Verification items for the finished model (mm, model axes). Face numbers are marked on the shaded views. A direction names the side the tool comes from. Round coordinates to 2 decimals unless told otherwise and drop trailing zeros. Order: outer loops, then holes, each group sorted by start corner. A loop starts at its lowest first (then second) coordinate and runs counter-clockwise, first axis right, second up. Notation, with made-up numbers: M -27,-23.5 L 26,-23.5 A38 cw 26,15.5 Z; hole C -9.75,-28.5 d3. An arc over 180 degrees is marked long. Return JSON: item names as keys, results as strings. Group by question number.
from build123d import *

# Parameters (mm, degrees)
F0_R      = 12.5
F1_DEPTH  = 40
F3_W      = 45
F3_H      = 200
F4_DEPTH  = 20
F5_W      = 35
F5_H      = 80
F6_DEPTH  = 25
F9_W      = 45
F9_H      = 10
F10_DEPTH = 1
F11_W     = 45
F11_H     = 10
F12_DEPTH = 1
F15_DEPTH = 2
F17_R     = 2.5
F18_DEPTH = 20.001


with BuildPart() as f1:
    # F0 (on Front) → F1 (new body)
    with BuildSketch(Plane.XZ):
        Circle(F0_R)
    extrude(amount=F1_DEPTH)

    # F3 (on offset) → F4 (join)
    with BuildSketch(Plane.XZ.offset(10)):
        Rectangle(F3_W, F3_H)
    extrude(amount=-F4_DEPTH)

    # F5 (on face) → F6 (cut)
    with BuildSketch(Plane(origin=(0, 10, 0), x_dir=(-1, 0, 0), z_dir=(0, 1, 0))):
        with Locations((0, 55)):
            Rectangle(F5_W, F5_H)
        with Locations((0, -55)):
            Rectangle(F5_W, F5_H)
    extrude(amount=-F6_DEPTH, mode=Mode.SUBTRACT)

    # F9 (on offset) → F10 (join)
    with BuildSketch(Plane.XY.offset(80)):
        with Locations((0, -5)):
            Rectangle(F9_W, F9_H)
    extrude(amount=-F10_DEPTH)

    # F11 (on offset) → F12 (join)
    with BuildSketch(Plane.XY.offset(-80)):
        with Locations((0, -5)):
            Rectangle(F11_W, F11_H)
    extrude(amount=F12_DEPTH)


with BuildPart() as f15:
    # F14 (on offset) → F15 (new body)
    with BuildSketch(Plane.XZ.offset(5)):
        with BuildLine():
            Line((-5, 88), (-5, 80))
            Line((-5, 80), (5, 80))
            Line((5, 80), (5, 88))
            ThreePointArc((5, 88), (0, 93), (-5, 88))
        make_face()
        with BuildLine():
            Line((5, -80), (-5, -80))
            Line((-5, -80), (-5, -88))
            ThreePointArc((-5, -88), (0, -93), (5, -88))
            Line((5, -88), (5, -80))
        make_face()
    extrude(amount=-F15_DEPTH)


with BuildPart() as f1_1:
    add(f1.part)

    # F16: union F15
    add(f15.part)

    # F17 (on face) → F18 (cut, through all)
    with BuildSketch(Plane.XZ.offset(10)):
        with Locations((0, -88)):
            Circle(F17_R)
        with Locations((0, 88)):
            Circle(F17_R)
    extrude(amount=-F18_DEPTH, mode=Mode.SUBTRACT)


solid = f1_1.part
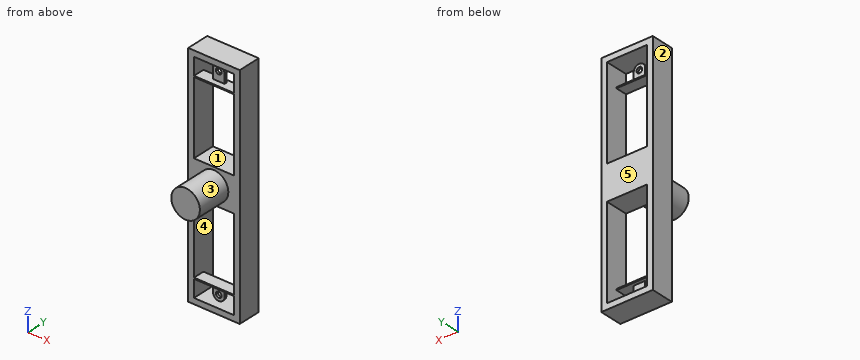
1. Cross-section at A-A (z = 60). Enter the section's corners in (x, y), plus the area to 3 significant figures.
2. Cross-section at D-D (x = 0). Give the number of separate pieces and of enclosed holes in the cut face, plus the area to 3 significant figures.
3. Thickness scan on line 1 along X through (y, z) = (3, 17); line 2 along Z through (x, y) = (-7.5, -5); line 3 along Y through (x, z) = (-19, 77). Record the ranges inside material, lowest first. Write a range as from..to.
4. Go/stop test with flat-tipped pins: pin 1 (8 mm diameter, centred on x = -1, z = 83.5, fed in from -Y); pin 2 (3 mm diameter, centred on x = 0, z = 88, fed in from +Y); pin 3 (8 mm diameter, centred on x = -1, z = -87, fed in from -Y); pin 4 (0.5 mm diameter, centred on x = -5.5, z = -79.5, fed in from +Y). Record where each tip stops, or that it passes through.
5. Cross-section at B-B (y = -7.5). Enter the section's corners in (x, z).
6. Access from +Z, -Z, +X, -X, +Y, -Y to the whole of each face (thin tool, end or side, straight path). Record for the marked faces 1 and 2.
7. Cross-section at C-C (z = 0). Enter the section's corners in (x, y), plus the area to 3 significant figures.
8. Draft check along X on the marked faces 3, 4 and 5. Enter one of: +X half, -X half, draft (parallel to the pull), parting line (faces both ways), or undercut.
Computed:
{
 "1": {"outline": "M -22.5,-10 L -17.5,-10 L -17.5,10 L -22.5,10 Z; M 17.5,-10 L 22.5,-10 L 22.5,10 L 17.5,10 Z", "area": "200 mm²"},
 "2": {"separate pieces": "7", "enclosed holes": "0", "area": "1,600 mm²"},
 "3": {"line 1": "x = -22.5..-17.5, 17.5..22.5", "line 2": "z = -100..-95, -80..-79, -15..15, 79..80, 95..100", "line 3": "y = -10..10"},
 "4": {"pin 1": "stops at y = -10", "pin 2": "passes through", "pin 3": "stops at y = -5", "pin 4": "stops at y = 0"},
 "5": {"outline": "M -22.5,-100 L 22.5,-100 L 22.5,100 L -22.5,100 Z; hole M -17.5,-95 L 17.5,-95 L 17.5,-80 L -17.5,-80 Z; hole M -17.5,-79 L 17.5,-79 L 17.5,-15 L -17.5,-15 Z; hole M -17.5,15 L 17.5,15 L 17.5,79 L -17.5,79 Z; hole M -17.5,80 L 17.5,80 L 17.5,95 L -17.5,95 Z"},
 "6": {"face 1": "+Y, -Y", "face 2": "+Z, -Z, -X, +Y, -Y"},
 "7": {"outline": "M -22.5,-10 L -12.5,-10 L -12.5,-40 L 12.5,-40 L 12.5,-10 L 22.5,-10 L 22.5,10 L -22.5,10 Z", "area": "1,650 mm²"},
 "8": {"face 3": "parting line", "face 4": "undercut", "face 5": "draft"}
}
